Check sheet for the modelled part. Datum: model origin and axes. Units: mm. A direction names the side the tool comes from. Coordinates: 2 decimals unless noted, no trailing zeros. Loops run counter-clockwise (first coordinate to the right, second up) from the corner with the lowest first, then second, coordinate; pieces in that order, holes last. Notation, with made-up numbers: (65, 10.5) - (107, 10.5) arc R19 cw to (107, 25.5) - close; hole circle Ø2 at (54, -24.5). An arc over 180 degrees is marked (long way). Use a Markdown table: item, result. Add a question column.
1) Draft check along X on faces 4 (the cylindrical face through (31.83, 10.02, 5.18)), 5 (the flat face through (-1, -52.91, 3)), 6 (the flat face through (-40.815, 5, 6)). Enter one of: pulls with the +X half, pulls with the -X half, needs draft (parallel to the pull), parting line crosses it, or undercut.
2) Go/stop test with flat-tipped pins: P1, Ø1.2, axis at y = -1.5, z = 6.5, coming from the +X side (3 decimals); P2, Ø5, axis at y = 37.5, z = 7, coming from the -X side (3 decimals). Record where each tip stops, or that it passes through.
3) Sectioned sample at A-A, the plane x = 0. Enter the section's corners in (y, z), then the cut area to 3 significant figures.
4) Thickness scan on line 1 (Y direction, x = 0, z = 4.75); line 2 (X direction, y = 28.5, z = 1.25); line 3 (X direction, y = -16, z = 3.5) (3 decimals). Record the ranges inside material, lowest first.
5) Sectioned sample at B-B, the plane y = 37.5. Enter the section's corners in (x, z) (3 decimals).
6) Sectioned sample at C-C, the plane y = 0. Enter the section's corners in (x, z) (3 decimals), then the cut area to 3 significant figures.
7) Tool access check on faces 1 (the flat face through (-1, -42.08, 6)), 2 (the flat face through (40.815, 5, 6)), 3 (the flat face through (50.885, 0, 3)). Record the directions out of +Z, -Z, +X, -X, +Y, -Y that give a thin tool (end or side, any length) a straight path to the whole face; none if there is none.
from build123d import *

# Parameters (mm, degrees)
F0_W         = 101.77
F0_H         = 105.82
F0_R         = 33.37
F1_DEPTH     = 4.38
F2_W         = 81.63
F2_H         = 94.99
F2_R         = 33.37
F3_DEPTH     = 4.07
F4_R         = 2
F5_T1_DEPTH  = 7.38
F5_S5_W      = 2
F5_S5_H      = 2
F5_T6_DEPTH  = 2
F5_S11_W     = 2
F5_S11_H     = 2
F5_T12_DEPTH = 2


# Not quite as in the source:
# - a fillet or chamfer that OpenCascade refuses, or shapes differently, is made with other operations: its cross-section is extruded or revolved along the edge and cut away or added


with BuildPart() as f1:
    # F0 (on Top) → F1 (new body)
    with BuildSketch(Plane.XY):
        Rectangle(F0_W, F0_H)
        Circle(F0_R, mode=Mode.SUBTRACT)
    extrude(amount=F1_DEPTH)

    # F2 (on face) → F3 (join)
    with BuildSketch(Plane.XY.offset(4.38)):
        with Locations((0, 5.415)):
            Rectangle(F2_W, F2_H)
        Circle(F2_R, mode=Mode.SUBTRACT)
    extrude(amount=F3_DEPTH)

    # F4
    f4_edges = [f1.edges().sort_by_distance(p)[0] for p in [
        (-33.37, 0, 0),
        (-50.885, 0, 0),
        (0, -52.91, 0),
        (50.885, 0, 0),
    ]]
    fillet(f4_edges, radius=F4_R)

    # F5: fillet of radius 2 on 2 edges, made by hand

    # F5_s2 → F5_t1 (cut)
    with BuildSketch(Plane.XY.offset(2)):
        with BuildLine():
            ThreePointArc((48.885, -52.91), (50.2992135624, -52.3242135624), (50.885, -50.91))
            Line((50.885, -50.91), (50.885, -52.91))
            Line((50.885, -52.91), (48.885, -52.91))
        make_face()
        with BuildLine():
            ThreePointArc((-48.885, -52.91), (-50.2992135624, -52.3242135624), (-50.885, -50.91))
            Line((-50.885, -50.91), (-50.885, -52.91))
            Line((-50.885, -52.91), (-48.885, -52.91))
        make_face()
    extrude(amount=F5_T1_DEPTH, mode=Mode.SUBTRACT)


with BuildPart() as f5_tool4:
    # F5_s5 → F5_t6 (new body)
    with BuildSketch(Plane.XZ.offset(50.91)):
        with Locations((-49.885, 1)):
            Rectangle(F5_S5_W, F5_S5_H)
    extrude(amount=F5_T6_DEPTH)

    # F5_s7 → F5_t8 (revolve, cut)
    with BuildSketch(Plane(origin=(-48.885, -50.91, 2), x_dir=(0.7071067812, 0, 0.7071067812), z_dir=(0.7071067812, 0, -0.7071067812))):
        with BuildLine():
            ThreePointArc((0, -2), (2, 0), (0, 2))
            Line((0, 2), (0, -2))
        make_face()
    revolve(axis=Axis((-48.885, -50.91, 2), (0, -1, 0)), mode=Mode.SUBTRACT)


with BuildPart() as f1_1:
    add(f1.part)

    # F5_t3: cut F5_tool4
    add(f5_tool4.part, mode=Mode.SUBTRACT)


with BuildPart() as f5_tool10:
    # F5_s11 → F5_t12 (new body)
    with BuildSketch(Plane.XZ.offset(50.91)):
        with Locations((49.885, 1)):
            Rectangle(F5_S11_W, F5_S11_H)
    extrude(amount=F5_T12_DEPTH)

    # F5_s13 → F5_t14 (revolve, cut)
    with BuildSketch(Plane(origin=(48.885, -50.91, 2), x_dir=(-0.7071067812, 0, 0.7071067812), z_dir=(0.7071067812, 0, 0.7071067812))):
        with BuildLine():
            ThreePointArc((0, -2), (2, 0), (0, 2))
            Line((0, 2), (0, -2))
        make_face()
    revolve(axis=Axis((48.885, -50.91, 2), (0, -1, 0)), mode=Mode.SUBTRACT)


with BuildPart() as f1_2:
    add(f1_1.part)

    # F5_t9: cut F5_tool10
    add(f5_tool10.part, mode=Mode.SUBTRACT)


solid = f1_2.part
Solved:
| question | item | result |
|---|---|---|
| 1 | face 4 | undercut |
| 1 | face 5 | needs draft |
| 1 | face 6 | pulls with the -X half |
| 2 | P1 | stops at x = 40.815 |
| 2 | P2 | stops at x = -40.815 |
| 3 | outline | (-52.91, 2) arc R2 ccw to (-50.91, 0) - (-35.37, 0) arc R2 ccw to (-33.37, 2) - (-33.37, 8.45) - (-42.08, 8.45) - (-42.08, 4.38) - (-52.91, 4.38) - close; (33.37, 2) arc R2 ccw to (35.37, 0) - (52.91, 0) - (52.91, 8.45) - (33.37, 8.45) - close |
| 3 | area | 284 mm2 |
| 4 | line 1 | y = -42.08 to -33.37, 33.37 to 52.91 |
| 4 | line 2 | x = -50.74 to -17.64, 17.64 to 50.74 |
| 4 | line 3 | x = -50.885 to -29.284, 29.284 to 50.885 |
| 5 | outline | (-50.885, 2) arc R2 ccw to (-48.885, 0) - (48.885, 0) arc R2 ccw to (50.885, 2) - (50.885, 4.38) - (40.815, 4.38) - (40.815, 8.45) - (-40.815, 8.45) - (-40.815, 4.38) - (-50.885, 4.38) - close |
| 6 | outline | (-50.885, 2) arc R2 ccw to (-48.885, 0) - (-35.37, 0) arc R2 ccw to (-33.37, 2) - (-33.37, 8.45) - (-40.815, 8.45) - (-40.815, 4.38) - (-50.885, 4.38) - close; (33.37, 2) arc R2 ccw to (35.37, 0) - (48.885, 0) arc R2 ccw to (50.885, 2) - (50.885, 4.38) - (40.815, 4.38) - (40.815, 8.45) - (33.37, 8.45) - close |
| 6 | area | 211 mm2 |
| 7 | face 1 | +Z, +X, -X, -Y |
| 7 | face 2 | +Z, +X, +Y, -Y |
| 7 | face 3 | +Z, -Z, +X, +Y, -Y |
